The model under review builds one solid part; all positions refer to its coordinate system, in mm. Face numbers are marked on the shaded views. A direction names the side the tool comes from. Round coordinates to 2 decimals unless told otherwise and drop trailing zeros. Write each loop counter-clockwise with the first axis right and the second up, starting at its lowest first coordinate (ties: lowest second). Pieces come first, ordered by that corner, then holes. Notation, with made-up numbers: (74, -29) -> (112, -29) arc R26 ccw to (112, -9) -> close; hole circle Ø5 at (-4, -22.5). An arc over 180 degrees is marked (long way). Use CSV: the item, a comma, the result in double quotes. Start each with the question number.
1) Take a section at C-C, the plane y = 150. Give the boundary of the cut face in (x, z).
2) Machinability: for the marked faces 1 and 2, which of the approach directions +Z, -Z, +X, -X, +Y, -Y give a long, thin tool a straight path to every point of the face, cutting with its end or side? Answer none if there is none.
3) Wall thickness on probe 1 along X at (y, z) = (227, 44); probe 2 along X at (y, z) = (307.5, 3.5): over which ranges is each line inside the solid? List them lowest first. Write a range as [from, to].
4) Take a section at A-A, the plane z = 15. Give the boundary of the cut face in (x, y).
5) Mouldability with a two-part tool opening along Z and no side actions: class the marked faces 3, 4 and 5 as released by +Z, released by -Z, zero draft, split by the parting line, or undercut.
6) Take a section at B-B, the plane x = 17. Give the boundary of the cut face in (y, z), then the cut area to 4 significant figures.
7) For pin 1 Ø4 at (y, z) = (173.5, 23) entering from -X; pin 2 Ø12 at (x, z) = (6, 17.5) entering from +Y, all flat-tipped, find the tip position at first contact; note any pin that passes through.
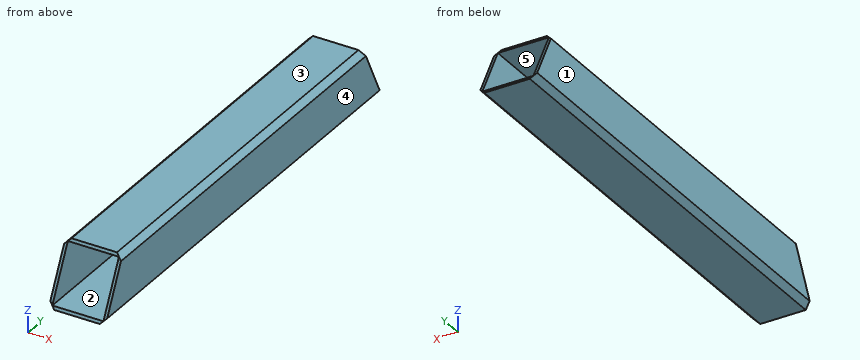
from build123d import *

# Parameters (mm, degrees)
SKETCH1_W           = 50
SKETCH1_H           = 400
BOSS_EXTRUDE2_DEPTH = 50
SKETCH2_W           = 45
SKETCH2_H           = 45
CUT_EXTRUDE1_DEPTH  = 407.201920232
CUT_EXTRUDE2_DEPTH  = 407.201920232
CHAMFER1_SIZE       = 5


with BuildPart() as part:
    # Sketch1 → Boss-Extrude2 (new body)
    with BuildSketch(Plane.XY):
        with Locations((25, 200)):
            Rectangle(SKETCH1_W, SKETCH1_H)
    extrude(amount=BOSS_EXTRUDE2_DEPTH)

    # Sketch2 → Cut-Extrude1 (cut, through all)
    with BuildSketch(Plane.XZ):
        with Locations((25, 25)):
            Rectangle(SKETCH2_W, SKETCH2_H)
    extrude(amount=-CUT_EXTRUDE1_DEPTH, mode=Mode.SUBTRACT)

    # Sketch3 → Cut-Extrude2 (cut, through all)
    with BuildSketch(Plane.ZY):
        Polygon((0, 400), (50, 400), (50, 375), align=None)
        Polygon((0, 0), (50, 0), (50, 25), align=None)
    extrude(amount=-CUT_EXTRUDE2_DEPTH, mode=Mode.SUBTRACT)

    # Chamfer1
    chamfer1_edges = [part.edges().sort_by_distance(p)[0] for p in [
        (0, 200, 50),
        (50, 200, 50),
        (50, 200, 0),
        (0, 200, 0),
    ]]
    chamfer(chamfer1_edges, length=CHAMFER1_SIZE - 0.0001)  # a hair under: the kernel refuses the full size


solid = part.part
Values found:
1,outline,"(0, 5) -> (5, 0) -> (45, 0) -> (50, 5) -> (50, 45) -> (45, 50) -> (5, 50) -> (0, 45) -> close; hole (2.5, 2.5) -> (47.5, 2.5) -> (47.5, 47.5) -> (2.5, 47.5) -> close"
2,face 1,"+Z, -Z, -X, +Y, -Y"
2,face 2,"+Y, -Y"
3,probe 1,"[0, 2.5], [47.5, 50]"
3,probe 2,"[1.5, 2.5], [47.5, 48.5]"
4,outline,"(0, 7.5) -> (2.5, 7.5) -> (2.5, 392.5) -> (0, 392.5) -> close; (47.5, 7.5) -> (50, 7.5) -> (50, 392.5) -> (47.5, 392.5) -> close"
5,face 3,"released by +Z"
5,face 4,"zero draft"
5,face 5,"undercut"
6,outline,"(0, 0) -> (400, 0) -> (398.75, 2.5) -> (1.25, 2.5) -> close; (23.75, 47.5) -> (376.25, 47.5) -> (375, 50) -> (25, 50) -> close"
6,area,"1,875 mm²"
7,pin 1,"x = 0"
7,pin 2,"y = 393.69"
